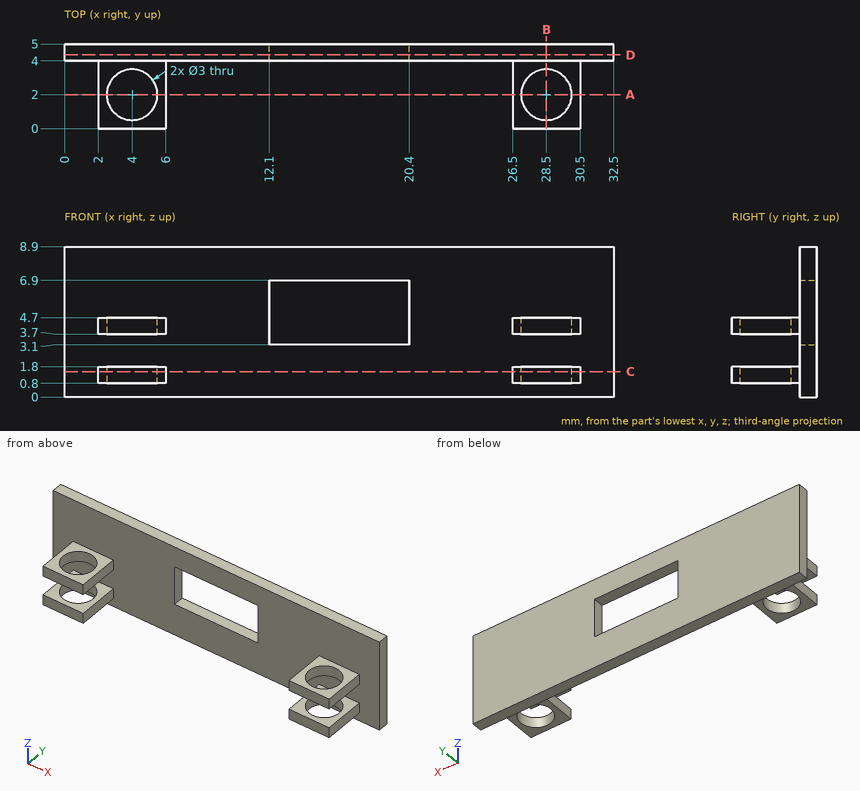
The drawing under review shows one solid part. Ordinate dimensions are in mm from its lowest x, y, z. Round coordinates to 2 decimals unless told otherwise and drop trailing zeros. Order: outer loops, then holes, each group sorted by start corner. A loop starts at its lowest first (then second) coordinate and runs counter-clockwise, first axis right, second up. Notation, with made-up numbers: (56.25, 85.25) - (112.25, 85.25) arc R21 ccw to (112.25, 115.25) - close; hole circle Ø10 at (75.5, 86.5). An arc over 180 degrees is marked (long way). Return JSON: item names as keys, results as strings.
Q1. Consider section B-B on x = 28.5. Write out the cut boundary in (y, z).
Computed values:
{"outline": "(0, 0.8) - (0.5, 0.8) - (0.5, 1.8) - (0, 1.8) - close; (0, 3.7) - (0.5, 3.7) - (0.5, 4.7) - (0, 4.7) - close; (3.5, 0.8) - (4, 0.8) - (4, 0) - (5, 0) - (5, 8.9) - (4, 8.9) - (4, 4.7) - (3.5, 4.7) - (3.5, 3.7) - (4, 3.7) - (4, 1.8) - (3.5, 1.8) - close"}
Q2. Wall thickness on L1, parallel to X at y = 2, z = 1.2; L2, parallel to Z at x = 2.5, y = 0.3; L3, parallel to Y at x = 28.5, z = 1.2: over which ranges is each line inside the solid? List them lowest first. Write a range as [from, to].
Computed values:
{"L1": "x = [2, 2.5], [5.5, 6], [26.5, 27], [30, 30.5]", "L2": "z = [0.8, 1.8], [3.7, 4.7]", "L3": "y = [0, 0.5], [3.5, 5]"}
Q3. Consider section D-D on y = 4.35. Write out the cut boundary in (x, z).
Computed values:
{"outline": "(0, 0) - (32.5, 0) - (32.5, 8.9) - (0, 8.9) - close; hole (12.1, 3.1) - (20.4, 3.1) - (20.4, 6.9) - (12.1, 6.9) - close"}
Q4. For pin 1 Ø2 at (x, y) = (28.5, 1) entering from -Z; pin 2 Ø1.1 at (y, z) = (1, 4.5) entering from +X; pin 3 Ø0.5 at (y, z) = (1.5, 4.5) entering from -X, all flat-tipped, find the tip position at first contact; note any pin that passes through.
Computed values:
{"pin 1": "stops at z = 0.8", "pin 2": "stops at x = 30.5", "pin 3": "stops at x = 2"}
Q5. Consider section C-C on z = 1.5. Write out the cut boundary in (x, y), plus the area to 3 significant figures.
Computed values:
{"outline": "(0, 4) - (2, 4) - (2, 0) - (6, 0) - (6, 4) - (26.5, 4) - (26.5, 0) - (30.5, 0) - (30.5, 4) - (32.5, 4) - (32.5, 5) - (0, 5) - close; hole circle Ø3 at (4, 2); hole circle Ø3 at (28.5, 2)", "area": "50.4 mm2"}
Q6. Consider section A-A on y = 2. Give the number of separate pieces and of enclosed holes in the cut face, plus the area to 3 significant figures.
Computed values:
{"separate pieces": "8", "enclosed holes": "0", "area": "4.00 mm2"}
